```python
from build123d import *

# Parameters (mm, degrees)
F0_R     = 25
F1_DEPTH = 125
F2_R     = 14.5
F3_DEPTH = 10
F4_R     = 35
F5_DEPTH = 120
F6_W     = 29
F6_H     = 10
F7_DEPTH = 200


with BuildPart() as f1:
    # F0 (on Top) → F1 (new body)
    with BuildSketch(Plane.XY):
        Circle(F0_R)
    extrude(amount=F1_DEPTH)

    # F2 (on face) → F3 (join)
    with BuildSketch(Plane.XY.offset(125)):
        Circle(F2_R)
    extrude(amount=F3_DEPTH)

    # F4 (on face) → F5 (join)
    with BuildSketch(Plane.XY.offset(135)):
        Circle(F4_R)
    extrude(amount=F5_DEPTH)

    # F6 (on Right) → F7 (join)
    with BuildSketch(Plane.YZ):
        Polygon((-35, 255), (-35, 135), (-14.5, 135), (14.5, 135), (35, 135), (35, 255), align=None)
        with Locations((0, 130)):
            Rectangle(F6_W, F6_H)
        Polygon((14.5, 125), (-14.5, 125), (-25, 125), (-25, 0), (25, 0), (25, 125), align=None)
    extrude(amount=F7_DEPTH)


solid = f1.part
```
Could you check a few things on this model? Use its own coordinates, in mm. A direction names the side the tool comes from. Give positions to 0.01 mm unless a question says otherwise; leave off trailing zeros. Order: outer loops, then holes, each group sorted by start corner. A loop starts at its lowest first (then second) coordinate and runs counter-clockwise, first axis right, second up.
Q1. Suppose I cut it at A-A, the plane x = 45. Write out the boundary of the cut face in (y, z).
Q2. For faces 4 (the flat face through (99, 25, 62)), 5 (the flat face through (99, -25, 63)), 6 (the flat face through (99, 14.5, 130)), 7 (the cylindrical face through (-24.994, 0.55, 61.625)), 8 (the cylindrical face through (-14.496, 0.319, 129.93)), which set-ups out of +Z, -Z, +X, -X, +Y, -Y let a thin tool reach every point of the face, with its end or its side?
Q3. We'd pull the mould along Z, two halves only. Please class faces 1 (the flat face through (99, 35, 194)), 2 (the flat face through (86, 0, 0)), 3 (the flat face through (99, -14.5, 130)): +Z half, -Z half, draft (parallel to the pull), parting line (faces both ways), or undercut.
Q4. Suppose I cut it at D-D, the plane z = 43. Write out the boundary of the cut face in (x, y), and give its area (3 significant figures).
Q5. If I drill on line 1 along Z through (x, y) = (114, 17); line 2 along Y through (x, z) = (98.5, 55); line 3 along X through (y, z) = (8, 52), over which ranges is the centre line in solid material (lowest first)?
Q6. Suppose I cut it at B-B, the plane y = 0. Write out the boundary of the cut face in (x, z).
Q7. I'm going to push flat-ended pins straight in: P1, Ø5, axis at x = 112, z = 128, coming from the -Y side; P2, Ø3, axis at x = 38.5, z = 117.5, coming from the +Y side; P3, Ø8, axis at y = 2, z = 157, coming from the -X side. Where does each tip first touch, or does it pass through?
Q8. Suppose I cut it at C-C, the plane z = 174.5. Write out the boundary of the cut face in (x, y).
Solution:
1. outline: (-35, 135) - (-14.5, 135) - (-14.5, 125) - (-25, 125) - (-25, 0) - (25, 0) - (25, 125) - (14.5, 125) - (14.5, 135) - (35, 135) - (35, 255) - (-35, 255) - close
2. face 4: -Z, +X, -X, +Y
2. face 5: -Z, +X, -X, -Y
2. face 6: +X, -X, +Y
2. face 7: -Z, -X
2. face 8: -X
3. face 1: draft
3. face 2: -Z half
3. face 3: undercut
4. outline: (0, -25) - (200, -25) - (200, 25) - (0, 25) arc R25 ccw to start
4. area: 11,000 mm2
5. line 1: z = 0 to 125, 135 to 255
5. line 2: y = -25 to 25
5. line 3: x = -23.69 to 200
6. outline: (-35, 135) - (-14.5, 135) - (-14.5, 125) - (-25, 125) - (-25, 0) - (200, 0) - (200, 255) - (-35, 255) - close
7. P1: stops at y = -14.5
7. P2: stops at y = 25
7. P3: stops at x = -35
8. outline: (0, -35) - (200, -35) - (200, 35) - (0, 35) arc R35 ccw to start
